Read the model definition and answer for the solid it produces. Units are mm, in the model's axes. A direction names the side the tool comes from. Round coordinates to 2 decimals unless told otherwise and drop trailing zeros. Loops run counter-clockwise (first coordinate to the right, second up) from the corner with the lowest first, then second, coordinate; pieces in that order, holes last. Notation, with made-up numbers: (5, 86) - (41, 86) arc R18 cw to (41, 108) - close; hole circle Ø6 at (4.5, 37.25). An arc over 180 degrees is marked (long way). Use CSV: the item, a comma, the result in double quotes. Start each with the question number.
1. Find section A-A (x = -81). Give the vertices of the cut face in (y, z) (3 decimals).
2. A tool of negligible diameter and unlimited length cuts with its end or side. For faces 4 (the flat face through (-114.808, -13, 77)), 5 (the flat face through (-2.54, -13, 77)), 6 (the flat face through (-59, -5, 0)), 7 (the flat face through (-58, -9.525, 137)), 8 (the flat face through (-58, -9.525, 22)), from which of +Z, -Z, +X, -X, +Y, -Y can it reach the whole face along a straight path? Write none if from no direction.
3. Consider line 1 along X through (y, z) = (-17.5, 82); line 2 along Y through (x, z) = (-13.5, 131.5) (3 decimals); line 3 along Z through (x, y) = (-94, -4). Determine where each line is inside the solid, lowest interval first.
4. Find section C-C (y = -22). Give the vertices of the cut face in (x, z).
5. Given pin 1 Ø14.5 at (y, z) = (-9.5, 79.5) entering from -X; pin 2 Ø1.5 at (x, z) = (-96, 129) entering from -Y (3 decimals); pin 3 Ø2 at (y, z) = (-6.5, 98.42) entering from -X; pin 4 Ø14.5 at (y, z) = (-8.5, 76) entering from +X, each flat-ended and moving along its own axis, determine where each tip first touches the part or whether it passes through.
6. Determine the mould class of faces 1 (the cylindrical face through (-116.096, -18.054, 79.726)), 2 (the flat face through (-57.853, -13.847, 105.848)), 3 (the flat face through (-59, 0, 78)) for opening direction Z: +Z half, -Z half, draft (parallel to the pull), parting line (faces both ways), or undercut.
7. Find section B-B (z = 29). Give the vertices of the cut face in (x, y) (3 decimals), and give its area (3 significant figures).
from build123d import *

# Parameters (mm, degrees)
SKETCH1_W           = 117.348
SKETCH1_H           = 38.1
BOSS_EXTRUDE1_DEPTH = 158.75
SKETCH2_R           = 1.35255
CUT_EXTRUDE1_DEPTH  = 152.4
SKETCH3_R           = 6.477
CUT_EXTRUDE4_DEPTH  = 154.686
SKETCH4_R           = 11.557
CUT_EXTRUDE5_DEPTH  = 2.54
CUT_EXTRUDE6_DEPTH  = 254
CHAMFER1_SIZE       = 6.35
FILLET1_R           = 10
FILLET2_R           = 2.54


with BuildPart() as part:
    # Sketch1 → Boss-Extrude1 (new body)
    with BuildSketch(Plane.XY):
        with Locations((-58.674, -19.05)):
            Rectangle(SKETCH1_W, SKETCH1_H)
    extrude(amount=BOSS_EXTRUDE1_DEPTH)

    # Sketch2 → Cut-Extrude1 (cut)
    with BuildSketch(Plane(origin=(0, 0, 0), x_dir=(0, 0, -1), z_dir=(1, 0, 0))):
        with Locations(Location((-98.425, -6.5024, 0), (0, 0, 90))):
            Circle(SKETCH2_R)
        with BuildLine():
            ThreePointArc((-78.02245, -25.5524), (-78.418602723, -24.596002723), (-79.375, -24.19985))
            Line((-79.375, -24.19985), (-79.375, -26.90495))
            ThreePointArc((-79.375, -26.90495), (-78.418602723, -26.508797277), (-78.02245, -25.5524))
        make_face()
        with BuildLine():
            Line((-79.375, -26.90495), (-79.375, -24.19985))
            ThreePointArc((-79.375, -24.19985), (-80.72755, -25.5524), (-79.375, -26.90495))
        make_face()
        with Locations(Location((-60.325, -6.5024, 0), (0, 0, 90))):
            Circle(SKETCH2_R)
    extrude(amount=-CUT_EXTRUDE1_DEPTH, mode=Mode.SUBTRACT)

    # Sketch3 → Cut-Extrude4 (cut)
    with BuildSketch(Plane(origin=(0, 0, 0), x_dir=(0, 0, -1), z_dir=(1, 0, 0))):
        with Locations(Location((-79.375, -6.5024, 0), (0, 0, 90))):
            Circle(SKETCH3_R)
    extrude(amount=-CUT_EXTRUDE4_DEPTH, mode=Mode.SUBTRACT)

    # Sketch4 → Cut-Extrude5 (cut)
    with BuildSketch(Plane(origin=(0, 0, 0), x_dir=(0, 0, -1), z_dir=(1, 0, 0))):
        with Locations((-79.375, -6.5024)):
            Circle(SKETCH4_R)
    cut_extrude5 = extrude(amount=-CUT_EXTRUDE5_DEPTH, mode=Mode.SUBTRACT)

    # Mirror1: Cut-Extrude5 across plane
    add(cut_extrude5.mirror(Plane(origin=(-58.674, 0, 0), x_dir=(0, 0, 1), z_dir=(1, 0, 0))), mode=Mode.SUBTRACT)

    # Sketch5 → Cut-Extrude6 (cut)
    with BuildSketch(Plane(origin=(0, 0, 0), x_dir=(0, 0, -1), z_dir=(1, 0, 0))):
        with BuildLine():
            Line((-158.75, -9.525), (-104.775, -9.525))
            ThreePointArc((-104.775, -9.525), (-79.375, -30.327663184), (-53.975, -9.525))
            Line((-53.975, -9.525), (0, -9.525))
            Line((0, -9.525), (0, -59.754484856))
            Line((0, -59.754484856), (-158.75, -59.754484856))
            Line((-158.75, -59.754484856), (-158.75, -9.525))
        make_face()
    extrude(amount=-CUT_EXTRUDE6_DEPTH, mode=Mode.SUBTRACT)

    # Chamfer1
    # the kernel refuses this chamfer: 6.35 mm, written as the material it adds along each edge
    with BuildSketch(Plane(origin=(0, -9.525, 104.775), x_dir=(0, -0.938739264670919, -0.3446281952555571), z_dir=(-1, 0, 0))) as chamfer1_piece_1:
        with BuildLine():
            Line((7.921952063, 0), (-CHAMFER1_SIZE * 0.344628195256, CHAMFER1_SIZE * 0.938739264671))
            Line((-CHAMFER1_SIZE * 0.344628195256, CHAMFER1_SIZE * 0.938739264671), (0, 0))
            ThreePointArc((0, 0), (4.071956682, 0.304341963), (7.921952063, 0))
        make_face()
    extrude(amount=117.348)
    with BuildSketch(Plane(origin=(0, -9.525, 53.975), x_dir=(0, 0, -1), z_dir=(-1, 0, 0))) as chamfer1_piece_2:
        with BuildLine():
            Line((CHAMFER1_SIZE, 0), (-2.730128042, 7.436647454))
            ThreePointArc((-2.730128042, 7.436647454), (-1.117613332, 3.927390442), (0, 0))
            Line((0, 0), (CHAMFER1_SIZE, 0))
        make_face()
    extrude(amount=117.348)

    # Fillet1
    fillet1_edges = [part.edges().sort_by_distance(p)[0] for p in [
        (-58.674, -9.525, 111.125),
        (-58.674, -16.961647454, 56.705128042),
        (-58.674, -16.961647454, 102.044871958),
        (-58.674, -9.525, 47.625),
    ]]
    fillet(fillet1_edges, radius=FILLET1_R)

    # Fillet2
    fillet2_edges = [part.edges().sort_by_distance(p)[0] for p in [
        (-117.348, -4.7625, 158.75),
        (-117.348, -4.7625, 0),
        (0, -4.7625, 0),
        (0, -4.7625, 158.75),
    ]]
    fillet(fillet2_edges, radius=FILLET2_R)


solid = part.part
Filled sheet:
1,outline,"(-18.247, 57.465) arc R10 cw to (-15.848, 55.345) - (-11.789, 50.389) arc R10 cw to (-9.525, 44.053) - (-9.525, 0) - (0, 0) - (0, 158.75) - (-9.525, 158.75) - (-9.525, 114.697) arc R10 cw to (-11.789, 108.361) - (-15.848, 103.405) arc R10 cw to (-18.247, 101.285) arc R25.908 ccw to start; hole circle Ø2.705 at (-25.552, 79.375); hole circle Ø12.954 at (-6.502, 79.375); hole circle Ø2.705 at (-6.502, 60.325); hole circle Ø2.705 at (-6.502, 98.425)"
2,face 4,"-X"
2,face 5,"+X"
2,face 6,"-Z, +X, -X, +Y, -Y"
2,face 7,"+Z, +X, -X, -Y"
2,face 8,"-Z, +X, -X, -Y"
3,line 1,"x = -114.81 to -2.54"
3,line 2,"y = -9.525 to 0"
3,line 3,"z = 0 to 73.4, 85.35 to 158.75"
4,outline,"(-117.35, 60.34) - (0, 60.34) - (0, 98.41) - (-117.35, 98.41) - close"
5,pin 1,"stops at x = -114.81"
5,pin 2,"stops at y = -9.525"
5,pin 3,"passes through"
5,pin 4,"stops at x = -2.54"
6,face 1,"undercut"
6,face 2,"+Z half"
6,face 3,"draft"
7,outline,"(-117.348, -9.525) - (0, -9.525) - (0, 0) - (-117.348, 0) - close"
7,area,"1,120 mm²"
